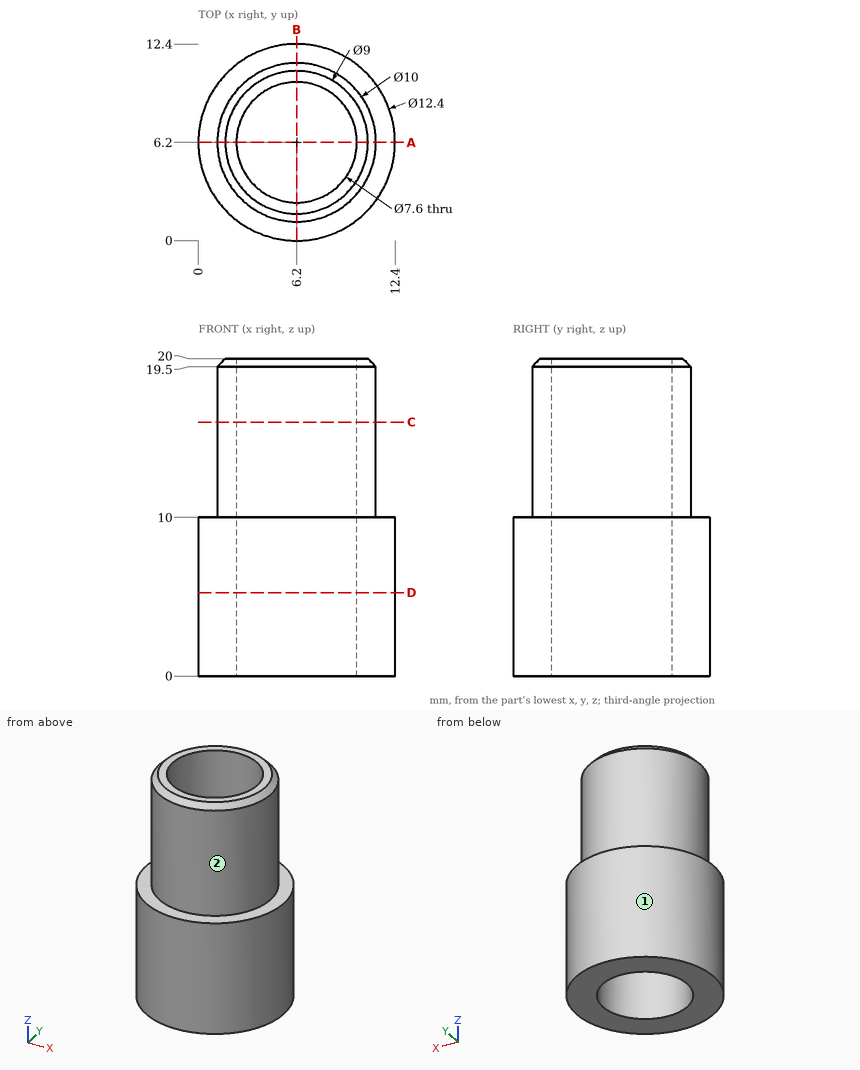
Study the drawing (mm; zero at the part's minimum x, y, z) and answer. A direction names the side the tool comes from. Coordinates: 2 decimals unless noted, no trailing zeros. Write each loop counter-clockwise with the first axis right and the second up, starting at its lowest first coordinate (ties: lowest second). Pieces come first, ordered by that corner, then holes. Notation, with made-up numbers: (54, -1.75) -> (76, -1.75) arc R16 cw to (76, 29.25) -> close; hole circle Ø6 at (-17.75, -36.5). An arc over 180 degrees is marked (long way). Write item = value, one per line.
(1) Section C-C on z = 16 is taken. Write down the section's boundary in (x, y).
From the geometry:
outline = circle Ø10 at (6.2, 6.2); hole circle Ø7.6 at (6.2, 6.2)
(2) Section A-A on y = 6.2 is taken. Write down the section's boundary in (x, z).
From the geometry:
outline = (0, 0) -> (2.4, 0) -> (2.4, 20) -> (1.7, 20) -> (1.2, 19.5) -> (1.2, 10) -> (0, 10) -> close; (10, 0) -> (12.4, 0) -> (12.4, 10) -> (11.2, 10) -> (11.2, 19.5) -> (10.7, 20) -> (10, 20) -> close
(3) Given pin 1 Ø6 at (y, z) = (2, 16) entering from -X; pin 2 Ø6 at (x, z) = (11, 2.5) entering from +Y; pin 3 Ø3 at (x, z) = (7, 15.5) entering from -Y, each flat-ended and moving along its own axis, determine where each tip first touches the part or whether it passes through.
From the geometry:
pin_1 = 1.35
pin_2 = 12.13
pin_3 = 1.2
(4) Straight lines are drawn through the part: L1, parallel to Y at x = 6.2, z = 12.75; L2, parallel to Y at x = 6.2, z = 7; L3, parallel to X at y = 9.25, z = 19. For each, find the intervals that lie inside material, in ascending order. Write a range as from..to.
From the geometry:
L1 = 1.2..2.4, 10..11.2
L2 = 0..2.4, 10..12.4
L3 = 2.24..3.93, 8.47..10.16
(5) Section D-D on z = 5.25 is taken. Write down the section's boundary in (x, y), plus the area to 3 significant figures.
From the geometry:
outline = circle Ø12.4 at (6.2, 6.2); hole circle Ø7.6 at (6.2, 6.2)
area = 75.4 mm2
(6) Which of the six approach directions +Z, -Z, +X, -X, +Y, -Y give full straight-line access (tool end or side, diameter ignored) to the marked faces 1 and 2?
From the geometry:
face_1 = +Z, -Z
face_2 = +Z
